Geometry: final body of the model. Coordinates: model frame, mm. A direction names the side the tool comes from. Round coordinates to 2 decimals unless told otherwise and drop trailing zeros. Loops run counter-clockwise (first coordinate to the right, second up) from the corner with the lowest first, then second, coordinate; pieces in that order, holes last. Notation, with made-up numbers: (10.5, 31.25) - (37.5, 31.25) arc R4 ccw to (37.5, 37.25) - close; hole circle Ø2 at (-21.5, 16.5). An arc over 180 degrees is marked (long way). Answer as a JSON object with one key per item and string values. Group by question number.
Item 1: Line query: line 1 (X direction, y = 2, z = 0); line 2 (Y direction, x = -46, z = 3); line 3 (Z direction, x = 45.5, y = -36). Output: solid intervals per line, ascending.
Item 2: Section B-B (z = 0). Return the cut outline in (x, y), plus the area to 3 significant figures.
Item 3: Section C-C (x = -3). Return the cut outline in (y, z), plus the area to 3 significant figures.
Item 4: Section A-A (y = -25.4). Return the cut outline in (x, z).
Item 5: Draft query along Y for faces 1 (the face through (-20.36, -21.54, -18.96)), 2 (the face through (22.47, -19.766, -18.961)), 3 (the face through (-1, -50.8, -19)), 4 (the face through (1, -28, -12.7)). Return one class per face: released by +Y, released by -Y, zero draft, split by the parting line, or undercut.
Item 6: First-contact query: pin 1 (6 mm diameter, centred on x = 39, y = -15.5, fed in from +Z); pin 2 (11.5 mm diameter, centred on x = 25.4, z = 0, fed in from -Y); pin 3 (8 mm diameter, centred on x = -9, z = -1, fed in from -Y). Flat tips, straight axial feed; report the tip coordinate or a pass-through.
Item 7: Section D-D (x = -26.5). Return the cut outline in (y, z).
Item 8: Reachability of faces 5 (the face through (-1, 12.7, 3)), 6 (the face through (-1, 0, 9)) from +Z, -Z, +X, -X, +Y, -Y: full face, straight path, thin tool, end or side. Return the list, or none.
Autodesk Fusion 360 part; units mm, degrees
sketch "Sketch1" plane through (0, 0, 0) normal (0, 1, 0) x (1, 0, 0)
  line L0 (50.8, 25.4) -> (-50.8, 25.4)
  line L1 (-50.8, 25.4) -> (-50.8, -25.4)
  line L2 (-50.8, -25.4) -> (50.8, -25.4)
  line L3 (50.8, -25.4) -> (50.8, 25.4)
  line L4 (0, 0) -> (25.4, 0) construction
  line L5 (0, 0) -> (-25.4, 0) construction
  circle A0 centre (-25.4, 0) radius 6.35
  circle A1 centre (25.4, 0) radius 6.35
  dimension "d3" = 101.6
  dimension "d4" = 50.8
  dimension "d5" = 25.4
  dimension "d7" = 12.7
  dimension "d8" = 12.7
extrude "Extrude1" add sketch "Sketch1" along normal blind 12.7 makes body 1
sketch "Sketch2" plane through (0, 0, 0) normal (0, -1, 0) x (1, 0, 0)
  circle A0 centre (-25.4, 0) radius 6.35
  circle A1 centre (25.4, 0) radius 6.35
  line L0 (50.8, -25.4) -> (50.8, 25.4)
  line L1 (50.8, 25.4) -> (-50.8, 25.4)
  line L2 (-50.8, 25.4) -> (-50.8, -25.4)
  line L3 (-50.8, -25.4) -> (50.8, -25.4)
  line L4 (-50.8, -25.4) -> (50.8, -25.4)
  line L5 (50.8, -25.4) -> (50.8, -12.7)
  line L6 (50.8, -12.7) -> (-50.8, -12.7)
  line L7 (-50.8, -12.7) -> (-50.8, -25.4)
  dimension "d11" = 101.6
  dimension "d12" = 12.7
extrude "Extrude2" add sketch "Sketch2" along normal blind 50.8 contours L0 L2 L3 L4 L5 L6 L7 bodies 1
sketch "Sketch3" plane through (0, 0, -12.7) normal (0, 0, 1) x (-1, 0, 0)
  line L0 (-50.8, 0) -> (50.8, 0)
  line L1 (50.8, 0) -> (50.8, 50.8)
  line L2 (50.8, 50.8) -> (-50.8, 50.8)
  line L3 (-50.8, 50.8) -> (-50.8, 0)
  line L4 (0, 0) -> (0, 50.8) construction
  line L5 (0, 25.4) -> (-25.4, 25.4) construction
  line L6 (0, 25.4) -> (25.4, 25.4) construction
  circle A0 centre (25.4, 25.4) radius 6.35
  circle A1 centre (-25.4, 25.4) radius 6.35
  dimension "d15" = 25.4
  dimension "d16" = 25.4
  dimension "d17" = 12.7
  dimension "d18" = 12.7
extrude "Extrude3" cut sketch "Sketch3" against normal blind 43.18 contours A0 | A1 bodies 1
fillet "Fillet1" radius 6.35 2 edges at (0, 0, -12.7) (0, 12.7, -25.4) on bodies 1
copy_body "Body->Comp1" bodies 1 removing the originals makes body 2 in component "Clamp/Mount Bracket"
component "Clamp/Mount Bracket" placed x (1, 0, 0) y (0, 1, 0) z (0, 0, 1) at (0, 0, 0)
equation "d7 = ( 1 / 2 ) * 1 in"
equation "d8 = ( 1 / 2 ) * 1 in"
equation "d9 = ( 1 / 2 ) * 1 in"
equation "d17 = ( 1 / 2 ) * 1 in"
equation "d18 = ( 1 / 2 ) * 1 in"
equation "d22 = ( 1 / 4 ) * 1 in"
Values:
{
 "1": {"line 1": "x = -50.8 to -31.75, -19.05 to 19.05, 31.75 to 50.8", "line 2": "y = 0 to 12.7", "line 3": "z = -25.4 to -12.7"},
 "2": {"outline": "(-50.8, 0) - (-31.75, 0) - (-31.75, 12.7) - (-50.8, 12.7) - close; (-19.05, 0) - (19.05, 0) - (19.05, 12.7) - (-19.05, 12.7) - close; (31.75, 0) - (50.8, 0) - (50.8, 12.7) - (31.75, 12.7) - close", "area": "968 mm^2"},
 "3": {"outline": "(-50.8, -25.4) - (6.35, -25.4) arc R6.35 ccw to (12.7, -19.05) - (12.7, 25.4) - (0, 25.4) - (0, -6.35) arc R6.35 cw to (-6.35, -12.7) - (-50.8, -12.7) - close", "area": "1,290 mm^2"},
 "4": {"outline": "(-50.8, -25.4) - (-31.75, -25.4) - (-31.75, -12.7) - (-50.8, -12.7) - close; (-19.05, -25.4) - (19.05, -25.4) - (19.05, -12.7) - (-19.05, -12.7) - close; (31.75, -25.4) - (50.8, -25.4) - (50.8, -12.7) - (31.75, -12.7) - close"},
 "5": {"face 1": "undercut", "face 2": "undercut", "face 3": "released by -Y", "face 4": "zero draft"},
 "6": {"pin 1": "stops at z = -12.7", "pin 2": "passes through", "pin 3": "stops at y = 0"},
 "7": {"outline": "(-50.8, -25.4) - (-31.65, -25.4) - (-31.65, -12.7) - (-50.8, -12.7) - close; (-19.15, -25.4) - (6.35, -25.4) arc R6.35 ccw to (12.7, -19.05) - (12.7, -6.25) - (0, -6.25) - (0, -6.35) arc R6.35 cw to (-6.35, -12.7) - (-19.15, -12.7) - close; (0, 6.25) - (12.7, 6.25) - (12.7, 25.4) - (0, 25.4) - close"},
 "8": {"face 5": "+Z, -Z, +X, -X, +Y", "face 6": "+Z, +X, -X, -Y"}
}
